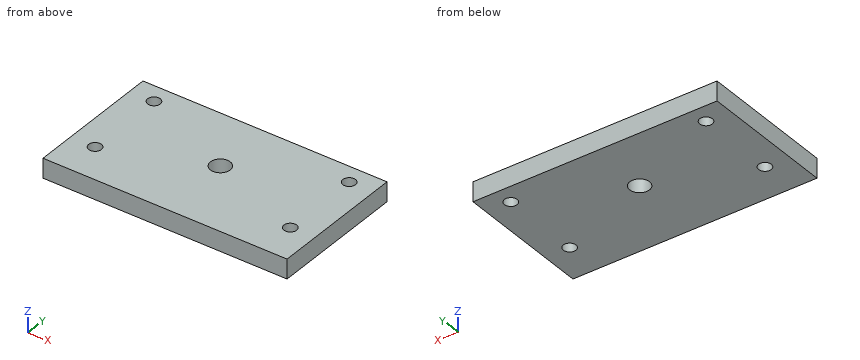
```python
from build123d import *

# Parameters (mm, degrees)
IZIM1_W                     = 100
IZIM1_H                     = 56
IZIM1_R                     = 4.05
Y_KSEKLIK_EKSTR_ZYON1_DEPTH = 8
IZIM3_R                     = 2.6
KES_EKSTR_ZYON2_DEPTH       = 10


with BuildPart() as part:
    # Çizim1 → Yükseklik-Ekstrüzyon1 (new body)
    with BuildSketch(Plane.XY):
        with Locations((7.377917159, -1.029772329)):
            Rectangle(IZIM1_W, IZIM1_H)
        with Locations((7.377917159, 1.970227671)):
            Circle(IZIM1_R, mode=Mode.SUBTRACT)
    extrude(amount=Y_KSEKLIK_EKSTR_ZYON1_DEPTH)

    # Çizim3 → Kes-Ekstrüzyon2 (cut)
    with BuildSketch(Plane.XY.offset(8)):
        with Locations((-32.622082841, 19.470227671)):
            Circle(IZIM3_R)
        with Locations((47.377917159, 19.470227671)):
            Circle(IZIM3_R)
        with Locations((47.377917159, -13.529772329)):
            Circle(IZIM3_R)
        with Locations((-32.622082841, -13.529772329)):
            Circle(IZIM3_R)
    extrude(amount=-KES_EKSTR_ZYON2_DEPTH, mode=Mode.SUBTRACT)


solid = part.part
```
Input: part model. Units: mm. Frame: model coordinates. Round coordinates to 2 decimals unless told otherwise and drop trailing zeros. Loops run counter-clockwise (first coordinate to the right, second up) from the corner with the lowest first, then second, coordinate; pieces in that order, holes last. Notation, with made-up numbers: (7, 79) -> (11, 79) arc R16 cw to (11, 91) -> close; hole circle Ø7 at (48, 64). An arc over 180 degrees is marked (long way). Write each question's results on one line, items separated by ' | '.
1. Section A-A (z = 4.25). Return loops of the section in (x, y), and give its area (3 significant figures).
Geometry results:
outline: (-42.62, -29.03) -> (57.38, -29.03) -> (57.38, 26.97) -> (-42.62, 26.97) -> close; hole circle Ø5.2 at (-32.62, -13.53); hole circle Ø5.2 at (-32.62, 19.47); hole circle Ø8.1 at (7.38, 1.97); hole circle Ø5.2 at (47.38, -13.53); hole circle Ø5.2 at (47.38, 19.47) | area: 5,460 mm2
2. Ray query, line 1 (Y direction, x = 7, z = 6.25); line 2 (X direction, y = -13, z = 5.5); line 3 (X direction, y = 20.5, z = 0.75). Return the intervals inside material, ascending. Write a range as from..to.
Geometry results:
line 1: -29.03..-2.06, 6..26.97 | line 2: -42.62..-35.17, -30.08..44.83, 49.92..57.38 | line 3: -42.62..-35.01, -30.23..44.99, 49.77..57.38
3. Section B-B (y = 0.5). Return loops of the section in (x, z).
Geometry results:
outline: (-42.62, 0) -> (3.6, 0) -> (3.6, 8) -> (-42.62, 8) -> close; (11.15, 0) -> (57.38, 0) -> (57.38, 8) -> (11.15, 8) -> close
4. First-contact query: P1, Ø3, axis at x = -32.62, y = 19.47, coming from the -Z side. Flat tip, straight axial feed; report the tip coordinate or a pass-through.
Geometry results:
P1: through
